Can you work these out from the model? Positions are in its coordinate system, mm. Face numbers are marked on the shaded views. A direction names the side the tool comes from. Coordinates: 2 decimals unless noted, no trailing zeros. Order: outer loops, then holes, each group sorted by start corner. A loop starts at its lowest first (then second) coordinate and runs counter-clockwise, first axis right, second up. Notation, with made-up numbers: (2.5, 19) -> (39.5, 19) arc R26 cw to (39.5, 49) -> close; hole circle Ø8 at (-38.5, 48). An arc over 180 degrees is marked (long way). Answer as CSV lines item,"result".
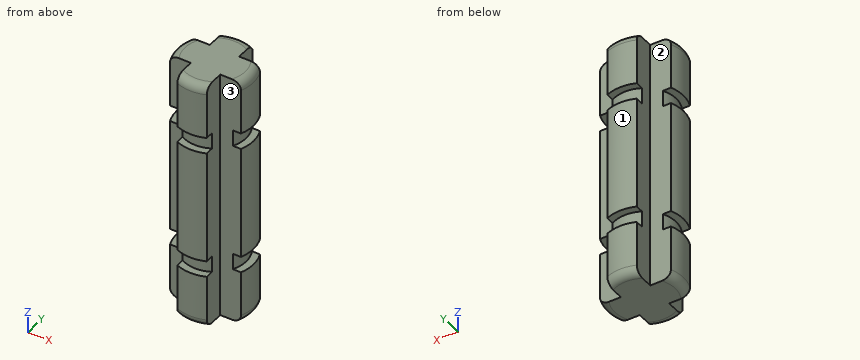
from build123d import *

# Parameters (mm, degrees)
BOSS_EXTRUDE1_DEPTH = 7.8
FILLET1_R           = 0.5
SIDE_START          = 3.5
SKETCH2_OUTSIDE_W   = 10.092
SKETCH2_OUTSIDE_H   = 10.092
SKETCH2_OUTSIDE_R   = 1.9
SIDE_CUT_DEPTH      = 1


with BuildPart() as part:
    # Sketch1 → Boss-Extrude1 (new, symmetric)
    with BuildSketch(Plane.XY):
        with BuildLine():
            Line((-0.9000000000000004, 0.9), (0.8999999999999999, 0.9000000000000002))
            Line((0.8999999999999998, 0.9000000000000004), (0.8999999999999998, 2.1708293346092873))
            ThreePointArc((0.8999999999999373, 2.170829334609268), (0.45883061344477144, 2.3047721076422936), (-1.386e-14, 2.3500000000000014))
            ThreePointArc((-1.386e-14, 2.3500000000000014), (-0.45883061344483045, 2.3047721076422825), (-0.9000000000000228, 2.170829334609233))
            Line((-0.9000000000000002, 2.170829334609226), (-0.9000000000000002, 0.8999999999999999))
        make_face()
        with BuildLine():
            Line((0.8999999999999998, 0.9000000000000004), (0.8999999999999998, -0.8999999999999999))
            Line((0.8999999999999999, -0.8999999999999998), (2.170829334609184, -0.8999999999999996))
            ThreePointArc((2.170829334609208, -0.9000000000000794), (2.304772107642276, -0.4588306134448533), (2.35, 2.9e-16))
            ThreePointArc((2.35, 8.7e-16), (2.3047721076422767, 0.4588306134448523), (2.1708293346092096, 0.9000000000000766))
            Line((2.170829334609186, 0.9000000000000004), (0.8999999999999999, 0.9000000000000002))
        make_face()
        with BuildLine():
            ThreePointArc((-0.9000000000000248, -2.1708293346092304), (-0.4588306134448299, -2.3047721076422807), (-1.13e-14, -2.3499999999999996))
            ThreePointArc((-1.13e-14, -2.3499999999999996), (0.45883061344477294, -2.304772107642292), (0.8999999999999382, -2.170829334609266))
            Line((0.8999999999999998, -2.1708293346092846), (0.8999999999999998, -0.8999999999999999))
            Line((0.8999999999999999, -0.8999999999999998), (-0.9000000000000004, -0.8999999999999999))
            Line((-0.9000000000000002, -0.8999999999999999), (-0.9000000000000002, -2.1708293346092233))
        make_face()
        with BuildLine():
            Line((-2.1708293346092815, -0.9000000000000001), (-0.9000000000000004, -0.8999999999999999))
            Line((-0.9000000000000002, -0.8999999999999999), (-0.9000000000000002, 0.8999999999999999))
            Line((-0.9000000000000004, 0.9), (-2.1708293346092815, 0.8999999999999999))
            ThreePointArc((-2.170829334609265, 0.8999999999999461), (-2.3047721076422913, 0.45883061344478315), (-2.350000000000001, 1.16e-15))
            ThreePointArc((-2.350000000000001, 1.16e-15), (-2.3047721076422913, -0.4588306134447819), (-2.170829334609264, -0.8999999999999455))
        make_face()
        Polygon((-0.9000000000000004, -0.8999999999999999), (0.8999999999999999, -0.8999999999999998), (0.8999999999999998, 0.9000000000000004), (-0.9000000000000004, 0.9), align=None)
    extrude(amount=BOSS_EXTRUDE1_DEPTH, both=True)

    # Fillet1
    fillet1_edges = [part.edges().sort_by_distance(p)[0] for p in [
        (-2.955e-14, 2.3500000000000014, 7.8),
        (2.3500000000000005, -9.3e-16, -7.8),
        (-2.982e-14, -2.3499999999999996, -7.8),
        (-2.350000000000001, 4.4e-16, -7.8),
        (-2.92e-14, 2.3500000000000014, -7.8),
        (-2.350000000000001, 2.2e-16, 7.8),
        (-2.943e-14, -2.3499999999999996, 7.8),
        (2.3499999999999996, -4.6e-16, 7.8),
    ]]
    fillet(fillet1_edges, radius=FILLET1_R)

    # Sketch2 outside → Side Cut (cut)
    with BuildSketch(Plane.XY.offset(SIDE_START)):
        Rectangle(SKETCH2_OUTSIDE_W, SKETCH2_OUTSIDE_H)
        Circle(SKETCH2_OUTSIDE_R, mode=Mode.SUBTRACT)
    side_cut = extrude(amount=SIDE_CUT_DEPTH, mode=Mode.SUBTRACT)

    # Mirror1: Side Cut across plane
    add(side_cut.mirror(Plane.XY), mode=Mode.SUBTRACT)


solid = part.part
Q1. Imagine slicing it at B-B (y = 0). List the corners of the cut face in (x, z) for me, and give its area (3 significant figures).
Solution:
outline,"(-2.35, -7.3) arc R0.5 ccw to (-1.85, -7.8) -> (1.85, -7.8) arc R0.5 ccw to (2.35, -7.3) -> (2.35, -4.5) -> (1.9, -4.5) -> (1.9, -3.5) -> (2.35, -3.5) -> (2.35, 3.5) -> (1.9, 3.5) -> (1.9, 4.5) -> (2.35, 4.5) -> (2.35, 7.3) arc R0.5 ccw to (1.85, 7.8) -> (-1.85, 7.8) arc R0.5 ccw to (-2.35, 7.3) -> (-2.35, 4.5) -> (-1.9, 4.5) -> (-1.9, 3.5) -> (-2.35, 3.5) -> (-2.35, -3.5) -> (-1.9, -3.5) -> (-1.9, -4.5) -> (-2.35, -4.5) -> close"
area,"71.3 mm2"
Q2. For P1, Ø2, axis at y = -1.5, z = -5, coming from the -X side; P2, Ø0.6, axis at y = 1.5, z = 3, coming from the -X side; P3, Ø0.6, axis at x = -1.5, z = 1, coming from the -Y side, each with a flat end and sliding along its axis, tell me the tip position at first contact or that it passes through.
Solution:
P1,"x = -2.3"
P2,"x = -0.9"
P3,"y = -0.9"
Q3. Imagine slicing it at A-A (z = 0.5). List the corners of the cut face in (x, y) for me, and give its area (3 significant figures).
Solution:
outline,"(-2.17, -0.9) -> (-0.9, -0.9) -> (-0.9, -2.17) arc R2.35 ccw to (0.9, -2.17) -> (0.9, -0.9) -> (2.17, -0.9) arc R2.35 ccw to (2.17, 0.9) -> (0.9, 0.9) -> (0.9, 2.17) arc R2.35 ccw to (-0.9, 2.17) -> (-0.9, 0.9) -> (-2.17, 0.9) arc R2.35 ccw to start"
area,"13.3 mm2"
Q4. Which directions (+Z, -Z, +X, -X, +Y, -Y) give clear straight access to the entire face, cutting with the end or side of a thin tool? Please do the marked faces 1, 2 and 3.
Solution:
face 1,"+Z, -Z, +Y"
face 2,"+Z, -Z, -X, +Y"
face 3,"+Z, -Z, +X, -Y"
Q5. If I drill on line 1 (X direction, y = -1.1, z = -3.75); line 2 (X direction, y = 0.1, z = 5.25), over which ranges is the centre line in solid material (lowest first)?
Solution:
line 1,"-0.9 to 0.9"
line 2,"-2.35 to 2.35"
Q6. Imagine slicing it at C-C (y = 1.2). List the corners of the cut face in (x, z) for me.
Solution:
outline,"(-0.9, -7.8) -> (0.9, -7.8) -> (0.9, 7.8) -> (-0.9, 7.8) -> close"
